Source: CAD feature listing. Evaluate the final solid. Frame: model axes, mm. Face numbers are marked on the shaded views. Give positions to 0.01 mm unless a question says otherwise; leave off trailing zeros. Order: outer loops, then holes, each group sorted by start corner. A loop starts at its lowest first (then second) coordinate and runs counter-clockwise, first axis right, second up. Notation, with made-up numbers: (33.25, 67) -> (57.25, 67) arc R29 ccw to (57.25, 94) -> close; hole circle Ø4 at (14.5, 88.5). An arc over 180 degrees is marked (long way). Answer in a Markdown table with one row per item.
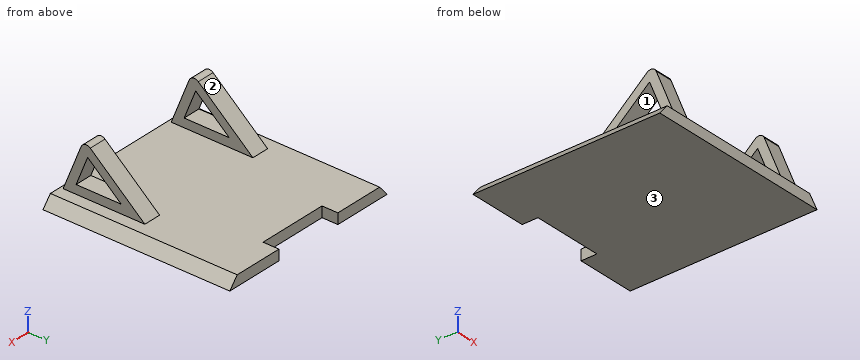
```python
from build123d import *

# Parameters (mm, degrees)
F3_DEPTH = 16
F4_W     = 12
F4_H     = 2.84
F5_DEPTH = 25
F1_DEPTH = 12.5
F6_DEPTH = 9.5


with BuildPart() as f3:
    # F2 (on Front) → F3 (new body, symmetric)
    with BuildSketch(Plane.XZ):
        Polygon((0, 1.8), (0, 0), (16, 0), (14.5, 1.8), align=None)
        Polygon((-16, 0), (0, 0), (0, 1.8), (-14.5, 1.8), align=None)
    extrude(amount=F3_DEPTH, both=True)

    # F4 (on Top) → F5 (cut)
    with BuildSketch(Plane.XY):
        with Locations((0, 14.7)):
            Rectangle(F4_W, F4_H)
    extrude(amount=F5_DEPTH, mode=Mode.SUBTRACT)

    # F0 (on Right) → F1 (join, symmetric)
    with BuildSketch(Plane.YZ):
        with BuildLine():
            Line((-12.426555, 9.427268), (-15.5, 1.8))
            Line((-15.5, 1.8), (-1.5, 1.8))
            Line((-1.5, 1.8), (-10.848235, 9.812773))
            ThreePointArc((-10.848235, 9.812773), (-11.736301, 10.024959), (-12.426555, 9.427268))
        make_face()
        Polygon((-13.278367, 3.3), (-11.295587, 8.220601), (-5.554886, 3.3), align=None, mode=Mode.SUBTRACT)
    extrude(amount=F1_DEPTH, both=True)

    # F0 (on Right) → F6 (cut, symmetric)
    with BuildSketch(Plane.YZ):
        with BuildLine():
            Line((-12.426555, 9.427268), (-15.5, 1.8))
            Line((-15.5, 1.8), (-1.5, 1.8))
            Line((-1.5, 1.8), (-10.848235, 9.812773))
            ThreePointArc((-10.848235, 9.812773), (-11.736301, 10.024959), (-12.426555, 9.427268))
        make_face()
        Polygon((-13.278367, 3.3), (-11.295587, 8.220601), (-5.554886, 3.3), align=None, mode=Mode.SUBTRACT)
        with BuildLine():
            Line((-15.5, 11.625779), (-15.5, 1.8))
            Line((-15.5, 1.8), (-12.426555, 9.427268))
            ThreePointArc((-12.426555, 9.427268), (-11.736301, 10.024959), (-10.848235, 9.812773))
            Line((-10.848235, 9.812773), (-13.849209, 12.385036))
            ThreePointArc((-13.849209, 12.385036), (-14.917857, 12.534292), (-15.5, 11.625779))
        make_face()
    extrude(amount=F6_DEPTH, both=True, mode=Mode.SUBTRACT)


solid = f3.part
```
(1) Section query A-A (y = 14.5). Return the cut outline in (x, z).
A:
| item | result |
|---|---|
| outline | (-16, 0) -> (-6, 0) -> (-6, 1.8) -> (-14.5, 1.8) -> close; (6, 0) -> (16, 0) -> (14.5, 1.8) -> (6, 1.8) -> close |
(2) Section query C-C (z = 8.75). Return the cut outline in (x, y).
A:
| item | result |
|---|---|
| outline | (-12.5, -12.7) -> (-9.5, -12.7) -> (-9.5, -9.61) -> (-12.5, -9.61) -> close; (9.5, -12.7) -> (12.5, -12.7) -> (12.5, -9.61) -> (9.5, -9.61) -> close |
(3) Section query B-B (x = -10). Return the cut outline in (y, z).
A:
| item | result |
|---|---|
| outline | (-16, 0) -> (16, 0) -> (16, 1.8) -> (-1.5, 1.8) -> (-10.85, 9.81) arc R1 ccw to (-12.43, 9.43) -> (-15.5, 1.8) -> (-16, 1.8) -> close; hole (-13.28, 3.3) -> (-5.55, 3.3) -> (-11.3, 8.22) -> close |
(4) Section query D-D (y = -7). Return the cut outline in (x, z).
A:
| item | result |
|---|---|
| outline | (-16, 0) -> (16, 0) -> (14.5, 1.8) -> (12.5, 1.8) -> (12.5, 3.3) -> (9.5, 3.3) -> (9.5, 1.8) -> (-9.5, 1.8) -> (-9.5, 3.3) -> (-12.5, 3.3) -> (-12.5, 1.8) -> (-14.5, 1.8) -> close; (-12.5, 4.54) -> (-9.5, 4.54) -> (-9.5, 6.51) -> (-12.5, 6.51) -> close; (9.5, 4.54) -> (12.5, 4.54) -> (12.5, 6.51) -> (9.5, 6.51) -> close |
(5) Pull-direction query (Z, two-part tool) for the marked faces 1, 2 and 3; classes: +Z half, -Z half, draft (parallel to the pull), parting line (faces both ways), or undercut.
A:
| item | result |
|---|---|
| face 1 | undercut |
| face 2 | +Z half |
| face 3 | -Z half |
(6) Ray query, probe 1 along X at (y, z) = (-11, 2.25); probe 2 along Z at (x, y) = (6, 10.5); probe 3 along Y at (x, z) = (4, 1.5). Return the intervals inside material, ascending.
A:
| item | result |
|---|---|
| probe 1 | x = -12.5 to -9.5, 9.5 to 12.5 |
| probe 2 | z = 0 to 1.8 |
| probe 3 | y = -16 to 13.28 |
(7) First-contact query: pin 1 Ø0.9 at (y, z) = (14.5, 0.5) entering from -X; pin 2 Ø4 at (y, z) = (-7, 5.5) entering from -X; pin 3 Ø3 at (x, y) = (9.5, 4) entering from -Z; pin 4 Ø2 at (x, z) = (1, 1) entering from +Y. Flat tips, straight axial feed; report the tip coordinate or a pass-through.
A:
| item | result |
|---|---|
| pin 1 | stops at x = -15.96 |
| pin 2 | stops at x = -12.5 |
| pin 3 | stops at z = 0 |
| pin 4 | stops at y = 13.28 |
